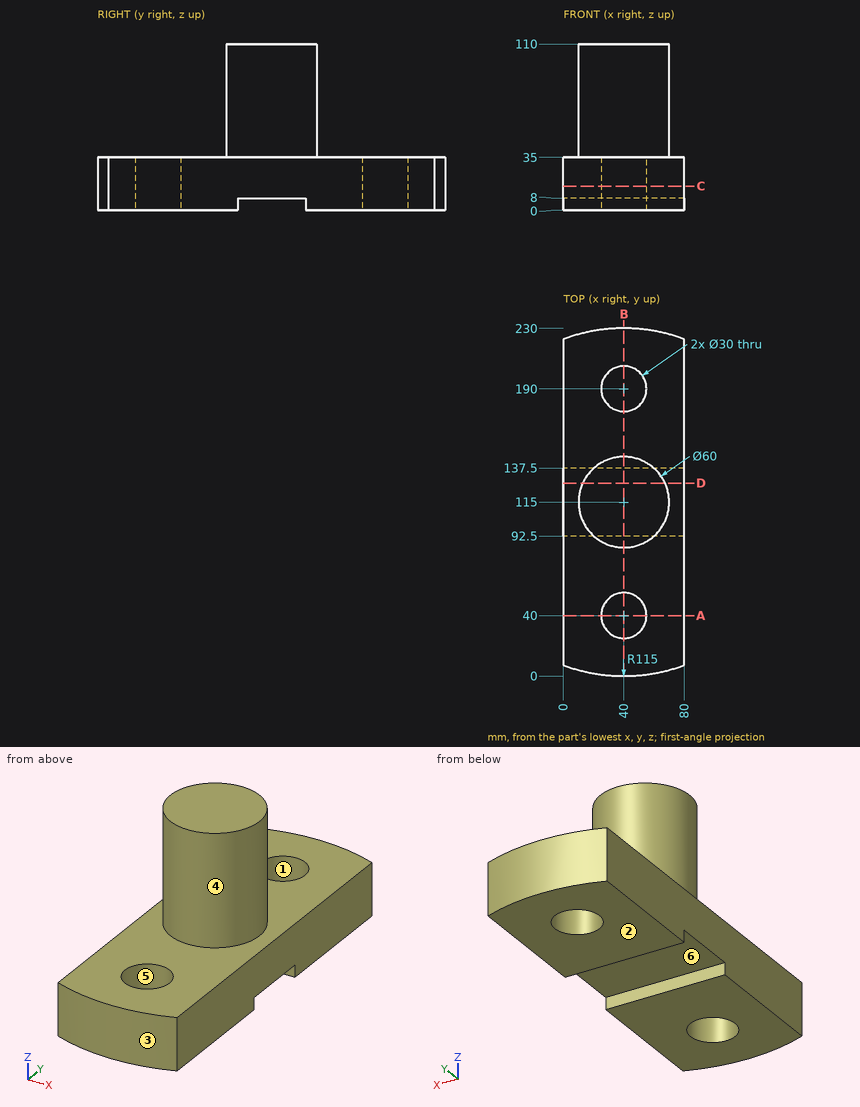
The figure shows three views and two pictorial views of one solid part (mm, origin at its lowest corner). Answer the questions. A direction names the side the tool comes from. Round coordinates to 2 decimals unless told otherwise and drop trailing zeros. Write each loop counter-clockwise with the first axis right and the second up, starting at its lowest first coordinate (ties: lowest second). Pieces come first, ordered by that corner, then holes. Notation, with made-up numbers: M 60.25,45 L 83.25,45 A10 cw 83.25,51 Z; hole C 8,25.5 d5. An arc over 180 degrees is marked long. Use a Markdown table: item, result.
1) The part is cut by section A-A (y = 40). Write down the section's boundary in (x, z).
Answers follow:
| item | result |
|---|---|
| outline | M 0,0 L 25,0 L 25,35 L 0,35 Z; M 55,0 L 80,0 L 80,35 L 55,35 Z |
2) Flat-ended cylindrical pins translate along their axes: pin 1 (1.5 mm diameter, centred on y = 106, z = 44.5, fed in from +X); pin 2 (4 mm diameter, centred on x = 19.5, y = 187, fed in from +Z); pin 3 (12 mm diameter, centred on x = 10, y = 104.5, fed in from -Z). Find the tip coordinate at first contact, or state that the pin passes through.
Answers follow:
| item | result |
|---|---|
| pin 1 | stops at x = 68.84 |
| pin 2 | stops at z = 35 |
| pin 3 | stops at z = 8 |
3) The part is cut by section B-B (x = 40). Write down the section's boundary in (y, z), plus the area to 3 significant figures.
Answers follow:
| item | result |
|---|---|
| outline | M 0,0 L 25,0 L 25,35 L 0,35 Z; M 55,0 L 92.5,0 L 92.5,8 L 137.5,8 L 137.5,0 L 175,0 L 175,35 L 145,35 L 145,110 L 85,110 L 85,35 L 55,35 Z; M 205,0 L 230,0 L 230,35 L 205,35 Z |
| area | 10,100 mm2 |
4) The part is cut by section D-D (y = 127.5). Write down the section's boundary in (x, z).
Answers follow:
| item | result |
|---|---|
| outline | M 0,8 L 80,8 L 80,35 L 67.27,35 L 67.27,110 L 12.73,110 L 12.73,35 L 0,35 Z |
5) The part is cut by section C-C (z = 16). Write down the section's boundary in (x, y), plus the area to 3 significant figures.
Answers follow:
| item | result |
|---|---|
| outline | M 0,7.18 A115 ccw 80,7.18 L 80,222.82 A115 ccw 0,222.82 Z; hole C 40,40 d30; hole C 40,190 d30 |
| area | 16,600 mm2 |
6) For a pull along X with two mould halves and no side action, classify the marked faces 1, 2 and 3 as pulls with the +X half, pulls with the -X half, needs draft (parallel to the pull), parting line crosses it, or undercut.
Answers follow:
| item | result |
|---|---|
| face 1 | undercut |
| face 2 | needs draft |
| face 3 | parting line crosses it |
7) Straight lines are drawn through the part: line 1 along Y through (x, z) = (30, 31); line 2 along Z through (x, y) = (42.5, 165); line 3 along Z through (x, y) = (45, 115.5). For each, find the intervals that lie inside material, in ascending order. Write a range as [from, to].
Answers follow:
| item | result |
|---|---|
| line 1 | y = [0.44, 28.82], [51.18, 178.82], [201.18, 229.56] |
| line 2 | z = [0, 35] |
| line 3 | z = [8, 110] |
8) A tool of negligible diameter and unlimited length cuts with its end or side. For the marked faces 4, 5 and 6, from which of +Z, -Z, +X, -X, +Y, -Y can it reach the whole face along a straight path? Write none if from no direction.
Answers follow:
| item | result |
|---|---|
| face 4 | +Z |
| face 5 | +Z, -Z |
| face 6 | -Z, +X, -X |
